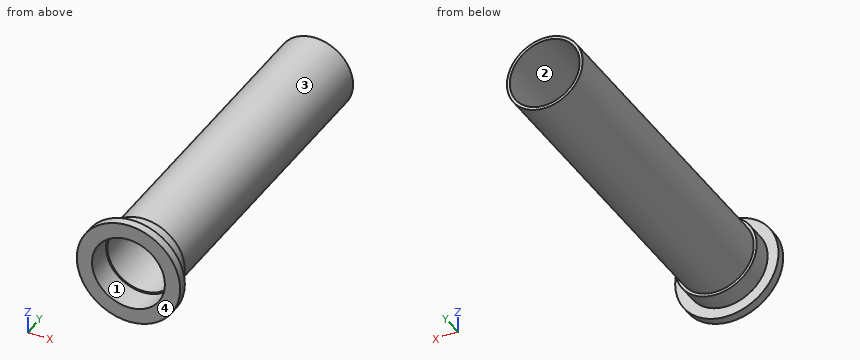
```python
from build123d import *

# Parameters (mm, degrees)
SKETCH2_R               = 41.275
SKETCH2_R_2             = 38.1
BASE_CYLINDER_DEPTH     = 381
SKETCH3_R               = 56.35625
SKETCH3_R_2             = 38.1
AFT_FLANGE_DEPTH        = 9.525
SKETCH34_R              = 39.75
TEMPERATUREINSERT_DEPTH = 28.575
SKETCH33_R              = 44.45
SKETCH33_R_2            = 41.275
CRITICALBOSS_DEPTH      = 22.225


with BuildPart() as part:
    # Sketch2 → Base Cylinder (new body)
    with BuildSketch(Plane(origin=(0, 0, 0), x_dir=(1, 0, 0), z_dir=(0, 1, 0))):
        Circle(SKETCH2_R)
        Circle(SKETCH2_R_2, mode=Mode.SUBTRACT)
    extrude(amount=BASE_CYLINDER_DEPTH)

    # Sketch3 → Aft Flange (add)
    with BuildSketch(Plane.XZ):
        Circle(SKETCH3_R)
        Circle(SKETCH3_R_2, mode=Mode.SUBTRACT)
    extrude(amount=-AFT_FLANGE_DEPTH)

    # Sketch34 → TemperatureInsert (cut)
    with BuildSketch(Plane.XZ):
        Circle(SKETCH34_R)
    extrude(amount=-TEMPERATUREINSERT_DEPTH, mode=Mode.SUBTRACT)

    # Sketch33 → CriticalBoss (add)
    with BuildSketch(Plane(origin=(0, 9.525, 0), x_dir=(1, 0, 0), z_dir=(0, 1, 0))):
        Circle(SKETCH33_R)
        Circle(SKETCH33_R_2, mode=Mode.SUBTRACT)
    extrude(amount=CRITICALBOSS_DEPTH)


solid = part.part
```
Input: part model. Units: mm. Frame: model coordinates. Face numbers are marked on the shaded views. Coordinates: 2 decimals unless noted, no trailing zeros. Write each loop counter-clockwise with the first axis right and the second up, starting at its lowest first coordinate (ties: lowest second). Pieces come first, ordered by that corner, then holes. Notation, with made-up numbers: M 30,57.5 L 79,57.5 A23 cw 79,74.5 Z; hole C 11.5,51 d6. An arc over 180 degrees is marked long. Use one line per item in the form item = value.
Q1. Draft query along X for the marked faces 1, 2, 3 and 4. Return one class per face: released by +X, released by -X, zero draft, split by the parting line, or undercut.
Answer below:
face_1 = undercut
face_2 = undercut
face_3 = split by the parting line
face_4 = zero draft
Q2. First-contact query: pin 1 (12 mm diameter, centred on y = 117.5, z = 6, fed in from +X) (3 decimals); pin 2 (6 mm diameter, centred on y = 128.5, z = 7.5, fed in from +X); pin 3 (1.5 mm diameter, centred on y = 235.5, z = -5, fed in from +X). Flat tips, straight axial feed; report the tip coordinate or a pass-through.
Answer below:
pin_1 = 41.275
pin_2 = 41.03
pin_3 = 41.06
Q3. Section A-A (x = 0). Return loops of the section in (y, z) (3 decimals).
Answer below:
outline = M 0,-56.356 L 9.525,-56.356 L 9.525,-44.45 L 31.75,-44.45 L 31.75,-41.275 L 381,-41.275 L 381,-38.1 L 28.575,-38.1 L 28.575,-39.75 L 0,-39.75 Z; M 0,39.75 L 28.575,39.75 L 28.575,38.1 L 381,38.1 L 381,41.275 L 31.75,41.275 L 31.75,44.45 L 9.525,44.45 L 9.525,56.356 L 0,56.356 Z
Q4. Section C-C (y = 57.5). Return loops of the section in (x, z) (3 decimals).
Answer below:
outline = C 0,0 d82.55; hole C 0,0 d76.2
Q5. Section B-B (z = 0). Return loops of the section in (x, y) (3 decimals), plus the area to 3 significant figures.
Answer below:
outline = M -56.356,0 L -39.75,0 L -39.75,28.575 L -38.1,28.575 L -38.1,381 L -41.275,381 L -41.275,31.75 L -44.45,31.75 L -44.45,9.525 L -56.356,9.525 Z; M 38.1,28.575 L 39.75,28.575 L 39.75,0 L 56.356,0 L 56.356,9.525 L 44.45,9.525 L 44.45,31.75 L 41.275,31.75 L 41.275,381 L 38.1,381 Z
area = 2,750 mm²
Q6. Material intervals for probe 1 along X at (y, z) = (116.5, 0) (3 decimals); probe 2 along Z at (x, y) = (2, 247); probe 3 along Y at (x, z) = (13, -45) (3 decimals), sorted ascending. Write a range as from..to.
Answer below:
probe_1 = -41.275..-38.1, 38.1..41.275
probe_2 = -41.23..-38.05, 38.05..41.23
probe_3 = 0..9.525
